```python
from build123d import *

# Parameters (mm, degrees)
SKETCH1_R               = 1.5
SKETCH1_W               = 182.468094358
SKETCH1_H               = 182.468094358
BOSS_EXTRUDE1_DEPTH     = 4
CUT_EXTRUDE1_DEPTH      = 10
CUT_EXTRUDE1_DEPTH_BACK = 10
SKETCH7_W               = 144.235193926
SKETCH7_H               = 4
FILLET1_R               = 4


with BuildPart() as part:
    # Sketch1 → Boss-Extrude1 (new body)
    with BuildSketch(Plane(origin=(0, 0, 0), x_dir=(1, 0, 0), z_dir=(0, 1, 0))):
        Polygon((154.855, -139.95), (165.325, -139.95), (165.325, 139.95), (154.855, 139.95), (154.855, 143.95), (138.875, 143.95), (138.875, 128.61722325), (132.375, 124.864446501), (125.875, 128.61722325), (125.875, 143.95), (-125.875, 143.95), (-125.875, 128.61722325), (-132.375, 124.864446501), (-138.875, 128.61722325), (-138.875, 143.95), (-154.855, 143.95), (-154.855, 139.95), (-165.325, 139.95), (-165.325, -139.95), (-154.855, -139.95), (-154.855, -143.95), (-138.875, -143.95), (-138.875, -128.61722325), (-132.375, -124.864446501), (-125.875, -128.61722325), (-125.875, -143.95), (125.875, -143.95), (125.875, -128.61722325), (132.375, -124.864446501), (138.875, -128.61722325), (138.875, -143.95), (154.855, -143.95), align=None)
        with Locations(Location((-147.795, -135.95, 0), (0, 0, 270))):
            Circle(SKETCH1_R, mode=Mode.SUBTRACT)
        with Locations(Location((-132.375, -119.95, 0), (0, 0, 270))):
            Circle(SKETCH1_R, mode=Mode.SUBTRACT)
        with Locations(Location((-119.795, -135.95, 0), (0, 0, 270))):
            Circle(SKETCH1_R, mode=Mode.SUBTRACT)
        with Locations(Location((-104.5, -113.5, 0), (0, 0, 270))):
            Circle(SKETCH1_R, mode=Mode.SUBTRACT)
        with Locations((0, -9)):
            Rectangle(SKETCH1_W, SKETCH1_H, mode=Mode.SUBTRACT)
        with Locations(Location((119.795, -135.95, 0), (0, 0, 270))):
            Circle(SKETCH1_R, mode=Mode.SUBTRACT)
        with Locations(Location((104.5, -113.5, 0), (0, 0, 270))):
            Circle(SKETCH1_R, mode=Mode.SUBTRACT)
        with Locations(Location((147.795, -135.95, 0), (0, 0, 270))):
            Circle(SKETCH1_R, mode=Mode.SUBTRACT)
        with Locations(Location((132.375, -119.95, 0), (0, 0, 270))):
            Circle(SKETCH1_R, mode=Mode.SUBTRACT)
        with Locations(Location((-104.5, 95.5, 0), (0, 0, 270))):
            Circle(SKETCH1_R, mode=Mode.SUBTRACT)
        with Locations(Location((-132.375, 119.95, 0), (0, 0, 270))):
            Circle(SKETCH1_R, mode=Mode.SUBTRACT)
        with Locations(Location((-147.795, 135.95, 0), (0, 0, 270))):
            Circle(SKETCH1_R, mode=Mode.SUBTRACT)
        with Locations(Location((-119.795, 135.95, 0), (0, 0, 270))):
            Circle(SKETCH1_R, mode=Mode.SUBTRACT)
        with Locations(Location((104.5, 95.5, 0), (0, 0, 270))):
            Circle(SKETCH1_R, mode=Mode.SUBTRACT)
        with Locations(Location((86.915968312, 117.1513625, 0), (0, 0, 270))):
            Circle(SKETCH1_R, mode=Mode.SUBTRACT)
        with Locations(Location((101.875, 117.1513625, 0), (0, 0, 270))):
            Circle(SKETCH1_R, mode=Mode.SUBTRACT)
        with Locations(Location((86.915968312, 133.95, 0), (0, 0, 270))):
            Circle(SKETCH1_R, mode=Mode.SUBTRACT)
        with Locations(Location((101.875, 133.95, 0), (0, 0, 270))):
            Circle(SKETCH1_R, mode=Mode.SUBTRACT)
        with Locations(Location((119.795, 135.95, 0), (0, 0, 270))):
            Circle(SKETCH1_R, mode=Mode.SUBTRACT)
        with Locations(Location((132.375, 119.95, 0), (0, 0, 270))):
            Circle(SKETCH1_R, mode=Mode.SUBTRACT)
        with Locations(Location((147.795, 135.95, 0), (0, 0, 270))):
            Circle(SKETCH1_R, mode=Mode.SUBTRACT)
    extrude(amount=BOSS_EXTRUDE1_DEPTH)

    # Sketch7 → Cut-Extrude1 (cut, two sides: drawn at the far end of the back side and taken through both)
    with BuildSketch(Plane.ZY.offset(-91.234047179).offset(-CUT_EXTRUDE1_DEPTH_BACK)):
        with Locations((9, 2)):
            Rectangle(SKETCH7_W, SKETCH7_H)
    extrude(amount=CUT_EXTRUDE1_DEPTH + CUT_EXTRUDE1_DEPTH_BACK, mode=Mode.SUBTRACT)

    # Fillet1
    fillet1_edges = [part.edges().sort_by_distance(p)[0] for p in [
        (91.234047179, 2, -63.117596963),
        (101.234047179, 2, -63.117596963),
        (91.234047179, 2, 81.117596963),
        (101.234047179, 2, 81.117596963),
        (91.234047179, 2, 100.234047179),
        (91.234047179, 2, -82.234047179),
        (-91.234047179, 2, -82.234047179),
        (-91.234047179, 2, 100.234047179),
    ]]
    fillet(fillet1_edges, radius=FILLET1_R)


solid = part.part
```
Can you work these out from the model? Positions are in its coordinate system, mm. Coordinates: 2 decimals unless noted, no trailing zeros. Loops run counter-clockwise (first coordinate to the right, second up) from the corner with the lowest first, then second, coordinate; pieces in that order, holes last. Notation, with made-up numbers: (-8.5, 8.25) - (32.5, 8.25) arc R31 ccw to (32.5, 40.25) - close; hole circle Ø4 at (52.25, -38.75). An arc over 180 degrees is marked (long way). Use a Markdown table: item, result.
Item 1: If I drill on probe 1 along X at (y, z) = (1.75, -95.5) (3 decimals); probe 2 along X at (y, z) = (1.85, -133.95) (3 decimals); probe 3 along Z at (x, y) = (97, 1), over which ranges is the centre line in solid material (lowest first)? Write a range as from..to.
Numbers:
| item | result |
|---|---|
| probe 1 | x = -165.325..-106, -103..103, 106..165.325 |
| probe 2 | x = -165.325..-138.875, -125.875..85.416, 88.416..100.375, 103.375..125.875, 138.875..165.325 |
| probe 3 | z = -143.95..-63.12, 81.12..143.95 |
Item 2: I want a section at C-C on y = 1.4. Give the number of separate pieces and of enclosed holes in the cut face, and give its area (3 significant figures).
Numbers:
| item | result |
|---|---|
| separate pieces | 1 |
| enclosed holes | 21 |
| area | 59,300 mm2 |
Item 3: Will this pin go through, and if not, where does the flat tip stop? pin 1 (1.2 mm diameter, centred on x = -161, y = 1.5, fed in from +Z).
Numbers:
| item | result |
|---|---|
| pin 1 | stops at z = 139.95 |
Item 4: I want a section at B-B on x = -78. Please give me the cut outline in (y, z), and give its area (3 significant figures).
Numbers:
| item | result |
|---|---|
| outline | (0, -143.95) - (4, -143.95) - (4, -82.23) - (0, -82.23) - close; (0, 100.23) - (4, 100.23) - (4, 143.95) - (0, 143.95) - close |
| area | 422 mm2 |
Item 5: I want a section at A-A on z = 60. Please give me the cut outline in (x, y) (3 decimals), and give its area (3 significant figures).
Numbers:
| item | result |
|---|---|
| outline | (-165.325, 0) - (-91.234, 0) - (-91.234, 4) - (-165.325, 4) - close; (101.234, 0) - (165.325, 0) - (165.325, 4) - (101.234, 4) - close |
| area | 553 mm2 |
